Part print with two shaded views. Sizes in mm from the minimum x, y, z corner. Coordinates: 2 decimals unless noted, no trailing zeros. Loops run counter-clockwise (first coordinate to the right, second up) from the corner with the lowest first, then second, coordinate; pieces in that order, holes last. Notation, with made-up numbers: (78.25, 10.5) -> (118.25, 10.5) arc R29 ccw to (118.25, 44.5) -> close; hole circle Ø4 at (-23.5, 32). An arc over 180 degrees is marked (long way). Answer as a JSON object with one key per item and string values. Group by question number.
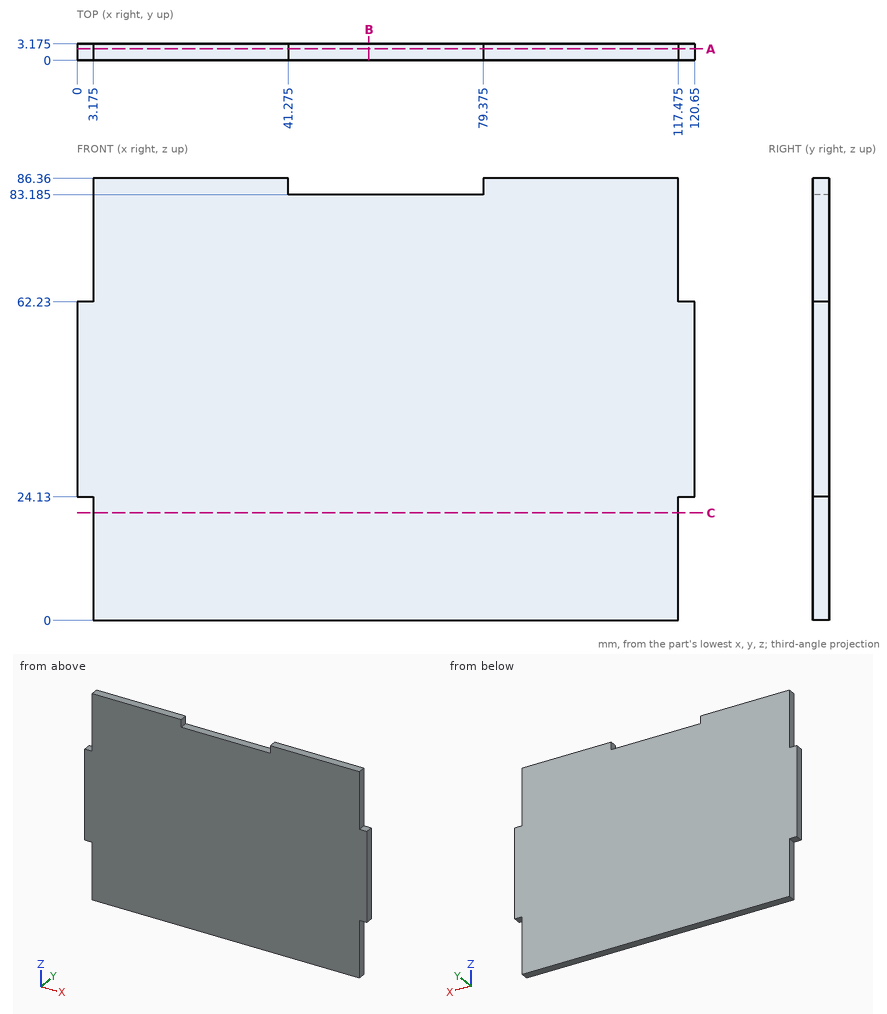
Item 1: Flat gauge pins, fed straight in: P1, Ø1, axis at y = 1, z = 84, coming from the +X side (3 decimals); P2, Ø1.6, axis at y = 2, z = 70, coming from the -X side (3 decimals). Where does each tip first touch, or does it go through?
Item 2: Drill centre lines: L1, parallel to Z at x = 42.5, y = 2.5 (3 decimals); L2, parallel to X at y = 0.8, z = 24 (3 decimals). Where is each one in solid material? Low to high.
Item 3: Band-saw the part on B-B, the plane x = 57. List the corners of the cut face in (y, z) (3 decimals), and give its area (3 significant figures).
Item 4: Band-saw the part on A-A, the plane y = 2.2. List the corners of the cut face in (x, z) (3 decimals), and give its area (3 significant figures).
Item 5: Band-saw the part on C-C, the plane z = 21. List the corners of the cut face in (x, y) (3 decimals), and give its area (3 significant figures).
Reply:
{
 "1": {"P1": "x = 117.475", "P2": "x = 3.175"},
 "2": {"L1": "0 to 83.185", "L2": "3.175 to 117.475"},
 "3": {"outline": "(0, 0) -> (3.175, 0) -> (3.175, 83.185) -> (0, 83.185) -> close", "area": "264 mm²"},
 "4": {"outline": "(0, 24.13) -> (3.175, 24.13) -> (3.175, 0) -> (117.475, 0) -> (117.475, 24.13) -> (120.65, 24.13) -> (120.65, 62.23) -> (117.475, 62.23) -> (117.475, 86.36) -> (79.375, 86.36) -> (79.375, 83.185) -> (41.275, 83.185) -> (41.275, 86.36) -> (3.175, 86.36) -> (3.175, 62.23) -> (0, 62.23) -> close", "area": "9,990 mm²"},
 "5": {"outline": "(3.175, 0) -> (117.475, 0) -> (117.475, 3.175) -> (3.175, 3.175) -> close", "area": "363 mm²"}
}
